For this review, use the dimensioned drawing (mm, ordinates from the lowest corner) and the shaded views. A direction names the side the tool comes from. Round coordinates to 2 decimals unless told otherwise and drop trailing zeros. Order: outer loops, then holes, each group sorted by start corner. A loop starts at its lowest first (then second) coordinate and runs counter-clockwise, first axis right, second up. Notation, with made-up numbers: M 79,-38.5 L 88,-38.5 A21 cw 88,-15.5 Z; hole C 1,70 d9. An arc over 180 degrees is marked long. Put each result on its own line as item: value.
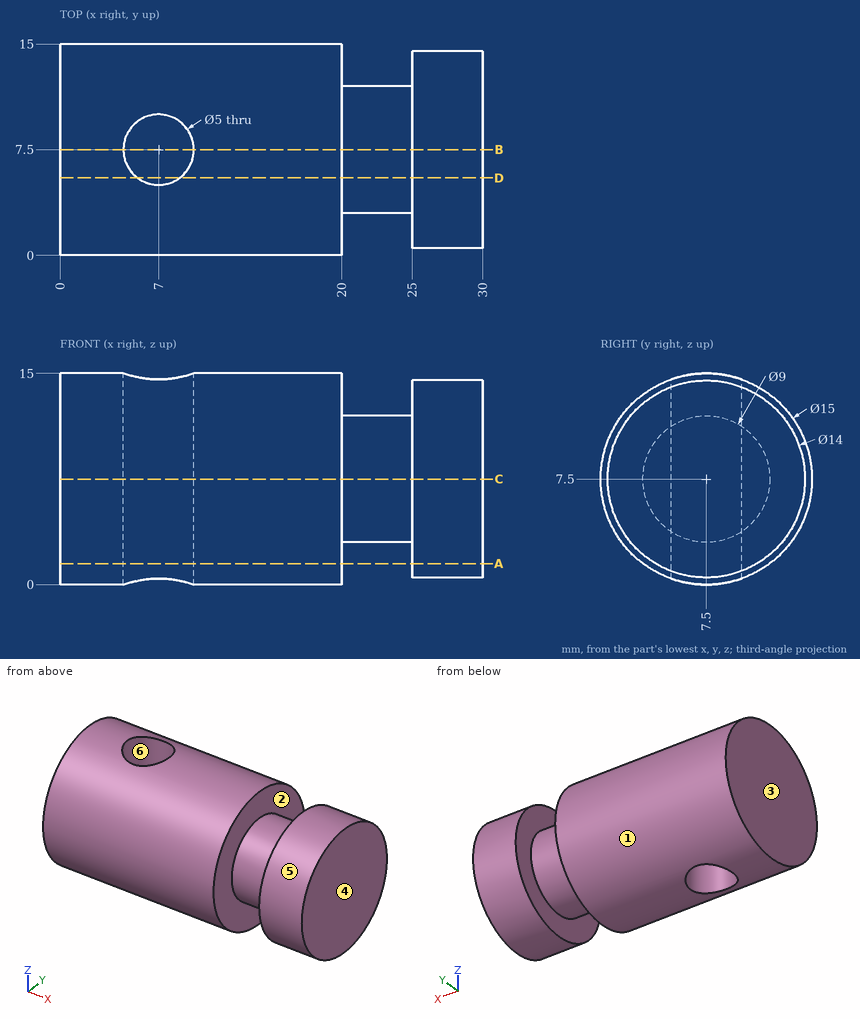
(1) Add section D-D on y = 5.5. Give the boundary of the cut face in (x, z).
A:
outline: M 0,0.27 L 5.5,0.27 L 5.5,14.73 L 0,14.73 Z; M 8.5,0.27 L 20,0.27 L 20,3.47 L 25,3.47 L 25,0.79 L 30,0.79 L 30,14.21 L 25,14.21 L 25,11.53 L 20,11.53 L 20,14.73 L 8.5,14.73 Z
(2) To check wall thickness, follow L1, parallel to Y at x = 7, z = 7.75; L2, parallel to X at y = 13, z = 10.75; L3, parallel to X at y = 6, z = 14.25. State the ranges of each line that lie inside material, in increasing order.
A:
L1: y = 0 to 5, 10 to 15
L2: x = 0 to 20, 25 to 30
L3: x = 0 to 5, 9 to 20, 25 to 30
(3) Insertion check: pin 1 Ø3 at (x, y) = (7, 7.5) entering from +Z; pin 2 Ø8 at (x, y) = (18.5, 4) entering from -Z; pin 3 Ø1.5 at (x, y) = (23.5, 6.5) entering from +Z; pin 4 Ø5 at (x, y) = (24.5, 4.5) entering from +Z. Each pin has a flat end and moves straight along its axis. Give the tip position at first contact, or say it passes through.
A:
pin 1: passes through
pin 2: stops at z = 0
pin 3: stops at z = 11.99
pin 4: stops at z = 14.48
(4) Draft analysis for pull direction X (two halves, no side actions). For the marked faces 3, 4, 5 and 6, state which applies: released by +X, released by -X, zero draft, split by the parting line, or undercut.
A:
face 3: released by -X
face 4: released by +X
face 5: zero draft
face 6: undercut
(5) For the marked faces 1 and 2, list the 3-axis set-ups (+Z, -Z, +X, -X, +Y, -Y) from which the entire face can be reached by the end or side of a thin tool; tool diameter is ignored.
A:
face 1: +X, -X
face 2: none
(6) Add section A-A on z = 1.5. Give the boundary of the cut face in (x, y).
A:
outline: M 0,3 L 20,3 L 20,12 L 0,12 Z; M 25,3.89 L 30,3.89 L 30,11.11 L 25,11.11 Z; hole C 7,7.5 d5
(7) Add section B-B on y = 7.5. Give the boundary of the cut face in (x, z).
A:
outline: M 0,0 L 4.5,0 L 4.5,15 L 0,15 Z; M 9.5,0 L 20,0 L 20,3 L 25,3 L 25,0.5 L 30,0.5 L 30,14.5 L 25,14.5 L 25,12 L 20,12 L 20,15 L 9.5,15 Z
(8) Add section C-C on z = 7.5. Give the boundary of the cut face in (x, y), then the cut area to 3 significant figures.
A:
outline: M 0,0 L 20,0 L 20,3 L 25,3 L 25,0.5 L 30,0.5 L 30,14.5 L 25,14.5 L 25,12 L 20,12 L 20,15 L 0,15 Z; hole C 7,7.5 d5
area: 395 mm2
